Geometry: see drawing. Coordinates: mm, zero at the bounding-box minimum. Coordinates: 2 decimals unless noted, no trailing zeros. Loops run counter-clockwise (first coordinate to the right, second up) from the corner with the lowest first, then second, coordinate; pieces in that order, holes last. Notation, with made-up numbers: (75, 78) - (100, 78) arc R9 ccw to (100, 87) - close; hole circle Ø6 at (2, 87.5). An arc over 180 degrees is marked (long way). Use a Markdown table: item, result. Add a question column.
1. Section query A-A on x = 5. Return the cut outline in (y, z).
2. Section query B-B on z = 12.5. Return the cut outline in (x, y).
3. Section query C-C on y = 21.5. Return the cut outline in (x, z).
4. Contact query for flat-ended pins moving along their axis: P1, Ø12, axis at x = 12.5, z = 22, coming from the +Y side; P2, Ø6, axis at x = 5, z = 12.5, coming from the +Y side; P3, Ø12, axis at x = 21, z = 19, coming from the +Y side. Output: stop coordinate, or through.
5. Draft query along X for the marked faces 1, 2 and 3. Return one class per face: released by +X, released by -X, zero draft, split by the parting line, or undercut.
6. Ray query, L1, parallel to X at y = 18, z = 13.25; L2, parallel to X at y = 1.3, z = 12.5 (1 decimal); L3, parallel to Z at x = 5, y = 2. Return the intervals inside material, ascending. Write a range as [from, to].
7. Section query D-D on x = 10. Return the cut outline in (y, z).
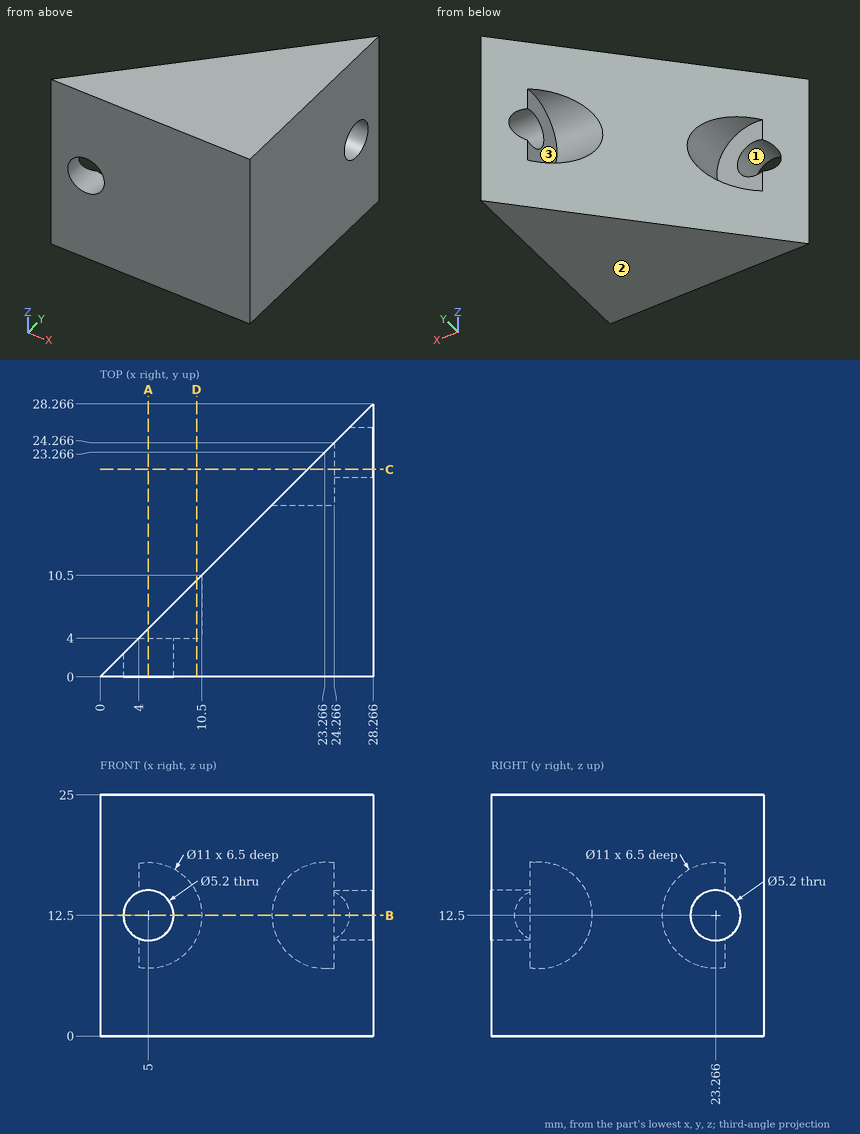
Resolved:
| question | item | result |
|---|---|---|
| 1 | outline | (0, 0) - (5, 0) - (5, 7) - (4, 7) - (4, 9.9) - (0, 9.9) - close; (0, 15.1) - (4, 15.1) - (4, 18) - (5, 18) - (5, 25) - (0, 25) - close |
| 2 | outline | (0, 0) - (2.4, 0) - (2.4, 2.4) - close; (7.6, 0) - (28.27, 0) - (28.27, 20.67) - (24.27, 20.67) - (24.27, 17.77) - (17.77, 17.77) - (10.5, 10.5) - (10.5, 4) - (7.6, 4) - close; (25.87, 25.87) - (28.27, 25.87) - (28.27, 28.27) - close |
| 3 | outline | (21.5, 0) - (28.27, 0) - (28.27, 10.59) - (24.27, 10.59) - (24.27, 7.29) - (21.5, 7.29) - close; (21.5, 17.71) - (24.27, 17.71) - (24.27, 14.41) - (28.27, 14.41) - (28.27, 25) - (21.5, 25) - close |
| 4 | P1 | y = 18.5 |
| 4 | P2 | y = 4 |
| 4 | P3 | y = 27 |
| 5 | face 1 | undercut |
| 5 | face 2 | zero draft |
| 5 | face 3 | released by -X |
| 6 | L1 | [24.27, 28.27] |
| 6 | L2 | [1.3, 2.4], [7.6, 28.3] |
| 6 | L3 | [0, 9.9], [15.1, 25] |
| 7 | outline | (0, 0) - (10, 0) - (10, 10.21) - (4, 10.21) - (4, 14.79) - (10, 14.79) - (10, 25) - (0, 25) - close |
